from build123d import *

# Parameters (mm, degrees)
SKETCH1_W           = 95.25
SKETCH1_H           = 95.25
BOSS_EXTRUDE1_DEPTH = 8.89
SKETCH2_OUTSIDE_W   = 124.25
SKETCH2_OUTSIDE_H   = 124.25
SKETCH2_OUTSIDE_W_2 = 95.25
SKETCH2_OUTSIDE_H_2 = 95.25
SKETCH2_OUTSIDE_R   = 2.38125
CUT_EXTRUDE2_DEPTH  = 9.89
SKETCH3_R           = 6.35
CUT_EXTRUDE3_DEPTH  = 4.445
SKETCH4_R           = 3.175
CUT_EXTRUDE4_DEPTH  = 5.445


with BuildPart() as part:
    # Sketch1 → Boss-Extrude1 (new body)
    with BuildSketch(Plane.XY):
        Rectangle(SKETCH1_W, SKETCH1_H)
    extrude(amount=BOSS_EXTRUDE1_DEPTH)

    # Sketch2 outside → Cut-Extrude2 (cut, through all)
    with BuildSketch(Plane.XY.offset(8.89)):
        Rectangle(SKETCH2_OUTSIDE_W, SKETCH2_OUTSIDE_H)
        Rectangle(SKETCH2_OUTSIDE_W_2, SKETCH2_OUTSIDE_H_2, mode=Mode.SUBTRACT)
        with Locations((-41.275, 41.275)):
            Circle(SKETCH2_OUTSIDE_R)
        with Locations((41.275, 41.275)):
            Circle(SKETCH2_OUTSIDE_R)
        with Locations((41.275, -41.275)):
            Circle(SKETCH2_OUTSIDE_R)
        with Locations((-41.275, -41.275)):
            Circle(SKETCH2_OUTSIDE_R)
    extrude(amount=-CUT_EXTRUDE2_DEPTH, mode=Mode.SUBTRACT)

    # Sketch3 → Cut-Extrude3 (cut)
    with BuildSketch(Plane.XY.offset(8.89)):
        with Locations((24.765, 29.845)):
            Circle(SKETCH3_R)
    extrude(amount=-CUT_EXTRUDE3_DEPTH, mode=Mode.SUBTRACT)

    # Sketch4 → Cut-Extrude4 (cut, through all)
    with BuildSketch(Plane.XY.offset(4.445)):
        with Locations((24.765, 29.845)):
            Circle(SKETCH4_R)
    extrude(amount=-CUT_EXTRUDE4_DEPTH, mode=Mode.SUBTRACT)


solid = part.part
Input: part model. Units: mm. Frame: model coordinates. A direction names the side the tool comes from. Coordinates: 2 decimals unless noted, no trailing zeros. Loops run counter-clockwise (first coordinate to the right, second up) from the corner with the lowest first, then second, coordinate; pieces in that order, holes last. Notation, with made-up numbers: (89, 84) -> (141, 84) arc R24 cw to (141, 116) -> close; hole circle Ø7 at (-2, 46). An arc over 180 degrees is marked (long way). One line per item, written item: value.
(1) Pin query (flat end, axial travel): pin 1 Ø4 at (x, y) = (23, 27.5) entering from +Z (3 decimals); pin 2 Ø5 at (x, y) = (24.765, 29.845) entering from +Z; pin 3 Ø7.5 at (x, y) = (-41.275, -41.275) entering from +Z. Return the tip coordinate at first contact, or that it passes through.
Answer below:
pin 1: stops at z = 4.445
pin 2: passes through
pin 3: stops at z = 8.89
(2) Cut plane A-A (z = 7). Give the number of separate pieces and of enclosed holes in the cut face, then the cut area to 3 significant figures.
Answer below:
separate pieces: 1
enclosed holes: 5
area: 8,870 mm2
(3) Ray query, line 1 along X through (y, z) = (-41, 2.5) (3 decimals); line 2 along X through (y, z) = (-42.5, 6.75) (3 decimals); line 3 along Y through (x, z) = (-40, 0.5) (3 decimals). Return the intervals inside material, ascending.
Answer below:
line 1: x = -47.625 to -43.64, -38.91 to 38.91, 43.64 to 47.625
line 2: x = -47.625 to -43.317, -39.233 to 39.233, 43.317 to 47.625
line 3: y = -47.625 to -43.286, -39.264 to 39.264, 43.286 to 47.625
(4) Set-up query: faces 1 (the face through (-47.625, -1, 4)), 2 (the face through (26, 33, 4.445)). Return all of +Z, -Z, +X, -X, +Y, -Y with unobstructed straight access to the full face (end or side cutting, diameter ignored); none if empty.
Answer below:
face 1: +Z, -Z, -X, +Y, -Y
face 2: +Z
(5) Cut plane B-B (y = 25). Output: boundary loops of the cut face in (x, z) (3 decimals).
Answer below:
outline: (-47.625, 0) -> (47.625, 0) -> (47.625, 8.89) -> (28.87, 8.89) -> (28.87, 4.445) -> (20.66, 4.445) -> (20.66, 8.89) -> (-47.625, 8.89) -> close
(6) Draft query along X for faces 3 (the face through (47.625, -1, 4)), 4 (the face through (-1, 47.625, 4)), 5 (the face through (-39.075, -42.187, 4.507)). Return one class per face: pulls with the +X half, pulls with the -X half, needs draft (parallel to the pull), parting line crosses it, or undercut.
Answer below:
face 3: pulls with the +X half
face 4: needs draft
face 5: undercut
